Autodesk Fusion 360 part; units mm, degrees
sketch "Sketch1" plane through (0, 0, 0) normal (0, 1, 0) x (1, 0, 0)
  line L0 (0, 0) -> (35, 0)
  line L1 (35, 0) -> (35, -35)
  line L2 (35, -35) -> (0, -35)
  line L3 (0, -35) -> (0, 0)
  line L4 (3.2, -3.2) -> (31.8, -3.2)
  line L5 (31.8, -3.2) -> (31.8, -31.8)
  line L6 (31.8, -31.8) -> (3.2, -31.8)
  line L7 (3.2, -31.8) -> (3.2, -3.2)
  dimension "d1" = 35
  dimension "d2" = 35
  dimension "d4" = 3.2
  dimension "d5" = 3.2
  dimension "d6" = 3.2
  dimension "d7" = 3.2
extrude "Extrude1" add sketch "Sketch1" along normal blind 30 makes body 1
sketch "Sketch2" plane through (0, 0, 35) normal (0, 0, 1) x (1, 0, 0)
  line L0 (0, 0) -> (35, 0)
  line L1 (35, 0) -> (35, 30)
  line L2 (35, 30) -> (0, 30)
  line L3 (0, 30) -> (0, 0)
  line L4 (5, 23.2) -> (15, 23.2)
  line L5 (15, 23.2) -> (15, 3.2)
  line L6 (15, 3.2) -> (5, 3.2)
  line L7 (5, 3.2) -> (5, 23.2)
  line L8 (20, 13.2) -> (30, 13.2)
  line L9 (30, 13.2) -> (30, 23.2)
  line L10 (30, 23.2) -> (20, 23.2)
  line L11 (20, 23.2) -> (20, 13.2)
  line L12 (0, 30) -> (-2.5, 30)
  line L13 (35, 30) -> (37.5, 30)
  line L14 (-2.5, 30) -> (17.5, 50)
  line L15 (17.5, 50) -> (37.5, 30)
  dimension "d10" = 3.2
  dimension "d11" = 5
  dimension "d12" = 20
  dimension "d13" = 10
  dimension "d14" = 10
  dimension "d15" = 10
  dimension "d16" = 13.2
  dimension "d17" = 5
  dimension "d39" = 2.5
  dimension "d40" = 2.5
  dimension "d41" = 20
  dimension "d42" = 20
extrude "Extrude2" add sketch "Sketch1" along normal blind 3.2 contours L4 L5 L6 L7 bodies 1
extrude "Extrude3" cut sketch "Sketch2" against normal blind 3.2 contours L4 L5 L6 L7 bodies 1
extrude "Extrude4" cut sketch "Sketch2" against normal blind 3.2 contours L8 L9 L10 L11 bodies 1
sketch "Sketch3" plane through (35, 0, 0) normal (1, 0, 0) x (0, 0, -1)
  line L0 (-35, 0) -> (0, 0)
  line L1 (0, 0) -> (0, 30)
  line L2 (0, 30) -> (-35, 30)
  line L3 (-35, 30) -> (-35, 0)
  line L4 (-22.5, 22.5) -> (-12.5, 22.5)
  line L5 (-12.5, 22.5) -> (-12.5, 12.5)
  line L6 (-12.5, 12.5) -> (-22.5, 12.5)
  line L7 (-22.5, 12.5) -> (-22.5, 22.5)
  line L8 (0, 0) -> (-35, 0)
  dimension "d24" = 10
  dimension "d25" = 10
  dimension "d26" = 12.5
  dimension "d27" = 12.5
extrude "Extrude5" cut sketch "Sketch3" against normal blind 35 contours L4 L5 L6 L7 bodies 1
sketch "Sketch4" plane through (0, 30, 0) normal (0, 1, 0) x (-1, 0, 0)
  line L0 (-31.8, 31.8) -> (-3.2, 31.8)
  line L1 (-3.2, 31.8) -> (-3.2, 3.2)
  line L2 (-3.2, 3.2) -> (-31.8, 3.2)
  line L3 (-31.8, 3.2) -> (-31.8, 31.8)
  line L4 (0, 35) -> (-35, 35)
  line L5 (-35, 35) -> (-35, 0)
  line L6 (-35, 0) -> (0, 0)
  line L7 (0, 0) -> (0, 35)
  line L8 (2.5, -2.5) -> (-37.5, -2.5)
  line L9 (-37.5, -2.5) -> (-37.5, 37.5)
  line L10 (-37.5, 37.5) -> (2.5, 37.5)
  line L11 (2.5, 37.5) -> (2.5, -2.5)
  line L12 (-30.8, 15.7) -> (-23.3, 15.7)
  line L13 (-23.3, 15.7) -> (-23.3, 8.2)
  line L14 (-23.3, 8.2) -> (-30.8, 8.2)
  line L15 (-30.8, 8.2) -> (-30.8, 15.7)
  dimension "d30" = 2.5
  dimension "d31" = 2.5
  dimension "d32" = 2.5
  dimension "d33" = 2.5
  dimension "d34" = 7.5
  dimension "d35" = 7.5
  dimension "d37" = 1
  dimension "d38" = 5
extrude "Extrude6" add sketch "Sketch2" along normal blind 2.5 separate body contours L2 L12 L13 L14 L15 makes body 2
extrude "Extrude7" add sketch "Sketch2" against normal blind 37.5 contours L2 L12 L13 L14 L15 bodies 1 2
extrude "Extrude8" add sketch "Sketch4" along normal blind 21 contours L12 L13 L14 L15 bodies 1
Work out the finished part from the listing and answer in its coordinate system (mm). A direction names the side the tool comes from. Give positions to 0.01 mm unless a question says otherwise; leave off trailing zeros. Write each loop counter-clockwise with the first axis right and the second up, starting at its lowest first coordinate (ties: lowest second). Pieces come first, ordered by that corner, then holes. Notation, with made-up numbers: (-21.75, -37.75) - (12.25, -37.75) arc R7 ccw to (12.25, -29.75) - close; hole circle Ø5 at (20, -34.5). An arc over 180 degrees is marked (long way). One line per item, written item: value. Start each with the question number.
1. Consider probe 1 along X at (y, z) = (16, 32.5); probe 2 along X at (y, z) = (23, 6). Determine where each line is inside the solid, lowest interval first.
2. For a pull along Z with two mould halves and no side action, classify faces 1 (the flat face through (35, 11, 17)), 2 (the flat face through (17, 38, 37.5)), 3 (the flat face through (33, 12.5, 17)) as +Z half, -Z half, draft (parallel to the pull), parting line (faces both ways), or undercut.
3. Find section B-B (z = 34). Write down the section's boundary in (x, y), then the cut area to 3 significant figures.
4. For faces 4 (the flat face through (0, 11, 18)), 5 (the flat face through (3.2, 10, 18)), 6 (the flat face through (2, 17, 22.5)), 7 (the flat face through (30.8, 44, 12)), determine the directions among +Z, -Z, +X, -X, +Y, -Y from which every point of the face is accessible in a straight line to the end or side of a thin tool.
5. Find section D-D (x = 12). Write down the section's boundary in (y, z).
6. Given pin 1 (1 mm diameter, centred on y = 15.5, z = 32.5, fed in from +X); pin 2 (10 mm diameter, centred on y = 36.5, z = 7.5, fed in from -X); pin 3 (10 mm diameter, centred on y = 6, z = 9, fed in from -X), each flat-ended and moving along its own axis, determine where each tip first touches the part or whether it passes through.
7. Find section C-C (y = 24). Write down the section's boundary in (x, z), then the cut area to 3 significant figures.
8. Find section A-A (y = 16.5). Write down the section's boundary in (x, z), then the cut area to 3 significant figures.
Geometry results:
1. probe 1: 0 to 5, 15 to 20, 30 to 35
1. probe 2: 0 to 3.2, 31.8 to 35
2. face 1: draft
2. face 2: +Z half
2. face 3: undercut
3. outline: (-2.5, 30) - (0, 30) - (0, 0) - (35, 0) - (35, 30) - (37.5, 30) - (17.5, 50) - close; hole (5, 3.2) - (15, 3.2) - (15, 23.2) - (5, 23.2) - close; hole (20, 13.2) - (30, 13.2) - (30, 23.2) - (20, 23.2) - close
3. area: 1,150 mm2
4. face 4: +Z, -Z, -X, -Y
4. face 5: none
4. face 6: +X, -X
4. face 7: +Z, -Z, +X, +Y
5. outline: (0, 0) - (30, 0) - (30, -2.5) - (44.5, -2.5) - (44.5, 37.5) - (30, 37.5) - (30, 35) - (23.2, 35) - (23.2, 31.8) - (30, 31.8) - (30, 3.2) - (3.2, 3.2) - (3.2, 35) - (0, 35) - close
6. pin 1: x = 35
6. pin 2: x = -1
6. pin 3: x = 0
7. outline: (0, 0) - (35, 0) - (35, 35) - (0, 35) - close; hole (3.2, 3.2) - (31.8, 3.2) - (31.8, 31.8) - (3.2, 31.8) - close
7. area: 407 mm2
8. outline: (0, 0) - (35, 0) - (35, 12.5) - (31.8, 12.5) - (31.8, 3.2) - (3.2, 3.2) - (3.2, 12.5) - (0, 12.5) - close; (0, 22.5) - (3.2, 22.5) - (3.2, 31.8) - (5, 31.8) - (5, 35) - (0, 35) - close; (15, 31.8) - (20, 31.8) - (20, 35) - (15, 35) - close; (30, 31.8) - (31.8, 31.8) - (31.8, 22.5) - (35, 22.5) - (35, 35) - (30, 35) - close
8. area: 279 mm2
